Geometry: final body of the model. Coordinates: model frame, mm. Face numbers are marked on the shaded views. A direction names the side the tool comes from. Give positions to 0.01 mm unless a question says otherwise; leave off trailing zeros. Write each loop counter-clockwise with the first axis right and the second up, starting at its lowest first coordinate (ties: lowest second). Pieces come first, ordered by that corner, then holes. Notation, with made-up numbers: (86.5, 64.5) -> (119.5, 64.5) arc R25 ccw to (119.5, 95.5) -> close; hole circle Ø3 at (32, 51). An arc over 180 degrees is marked (long way). Answer as a JSON object with one key per item and string values.
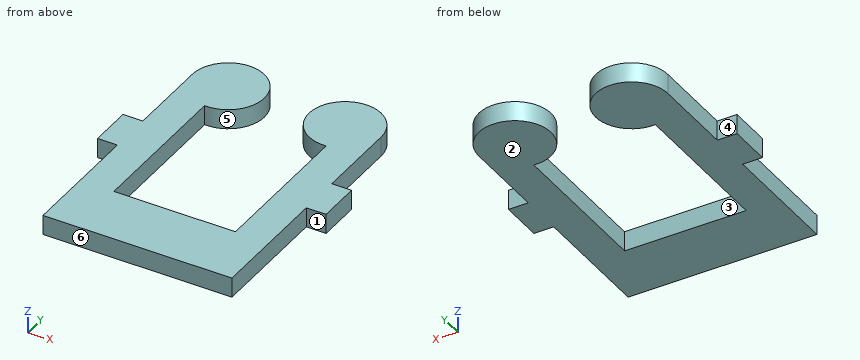
from build123d import *

# Parameters (mm, degrees)
BASE_START = 3
BASE_DEPTH = 3


with BuildPart() as part:
    # Sketch5 → Base (new body)
    with BuildSketch(Plane.XY.offset(9.55).offset(BASE_START)):
        with BuildLine():
            Line((9.2, 4.5), (-9.2, 4.5))
            Line((-9.2, 4.5), (-9.2, 27.686563585))
            ThreePointArc((-9.2, 27.686563585), (-4.864199201, 36.859644755), (-14.3, 33.13))
            Line((-14.3, 33.13), (-14.3, 20.5))
            Line((-14.3, 20.5), (-17.3, 20.5))
            Line((-17.3, 20.5), (-17.3, 14))
            Line((-17.3, 14), (-14.3, 14))
            Line((-14.3, 14), (-14.3, -5))
            Line((-14.3, -5), (14.3, -5))
            Line((14.3, -5), (14.3, 14))
            Line((14.3, 14), (17.3, 14))
            Line((17.3, 14), (17.3, 20.5))
            Line((17.3, 20.5), (14.3, 20.5))
            Line((14.3, 20.5), (14.3, 33.13))
            ThreePointArc((14.3, 33.13), (4.864199201, 36.859644755), (9.2, 27.686563585))
            Line((9.2, 27.686563585), (9.2, 4.5))
        make_face()
    extrude(amount=BASE_DEPTH)


solid = part.part
Q1. First-contact query: P1, Ø0.9, axis at y = 13, z = 13.5, coming from the -X side; P2, Ø0.9, axis at y = 6.5, z = 15, coming from the +X side; P3, Ø2, axis at x = -8.5, y = 15.5, coming from the -Z side; P4, Ø0.9, axis at x = -4, z = 13.5, coming from the +Y side. Flat tips, straight axial feed; report the tip coordinate or a pass-through.
Values:
{"P1": "x = -14.3", "P2": "x = 14.3", "P3": "z = 12.55", "P4": "y = 36.36"}
Q2. Cut plane D-D (x = 15). Return the cut outline in (y, z), and give its area (3 significant figures).
Values:
{"outline": "(14, 12.55) -> (20.5, 12.55) -> (20.5, 15.55) -> (14, 15.55) -> close", "area": "19.5 mm²"}
Q3. Cut plane C-C (z = 13.4). Return the cut outline in (x, y) (3 decimals), and give its area (3 significant figures).
Values:
{"outline": "(-17.3, 14) -> (-14.3, 14) -> (-14.3, -5) -> (14.3, -5) -> (14.3, 14) -> (17.3, 14) -> (17.3, 20.5) -> (14.3, 20.5) -> (14.3, 33.13) arc R5.455 ccw (long way) to (9.2, 27.687) -> (9.2, 4.5) -> (-9.2, 4.5) -> (-9.2, 27.687) arc R5.455 ccw (long way) to (-14.3, 33.13) -> (-14.3, 20.5) -> (-17.3, 20.5) -> close", "area": "747 mm²"}
Q4. Material intervals for L1, parallel to X at y = 18, z = 13.3; L2, parallel to X at y = 9.5, z = 14.9; L3, parallel to Y at x = 8.5, z = 13.6, sorted ascending. Write a range as from..to.
Values:
{"L1": "-17.3..-9.2, 9.2..17.3", "L2": "-14.3..-9.2, 9.2..14.3", "L3": "-5..4.5, 27.69..38.57"}
Q5. Set-up query: the marked faces 1, 2, 3 and 4. Return all of +Z, -Z, +X, -X, +Y, -Y with unobstructed straight access to the full face (end or side cutting, diameter ignored); none if empty.
Values:
{"face 1": "+Z, -Z, +X, -Y", "face 2": "-Z, +X, -X, +Y, -Y", "face 3": "+Z, -Z", "face 4": "+Z, -Z, -X, +Y"}
Q6. Mould query, pull axis X, two halves, no side actions, for the marked faces 5 and 6. Classes: pulls with the +X half, pulls with the -X half, needs draft (parallel to the pull), parting line crosses it, or undercut.
Values:
{"face 5": "undercut", "face 6": "needs draft"}
Q7. Cut plane A-A (y = 10). Return the cut outline in (x, z), and give its area (3 significant figures).
Values:
{"outline": "(-14.3, 12.55) -> (-9.2, 12.55) -> (-9.2, 15.55) -> (-14.3, 15.55) -> close; (9.2, 12.55) -> (14.3, 12.55) -> (14.3, 15.55) -> (9.2, 15.55) -> close", "area": "30.6 mm²"}
Q8. Cut plane B-B (x = -7). Return the cut outline in (y, z).
Values:
{"outline": "(-5, 12.55) -> (4.5, 12.55) -> (4.5, 15.55) -> (-5, 15.55) -> close; (28, 12.55) -> (38.26, 12.55) -> (38.26, 15.55) -> (28, 15.55) -> close"}
